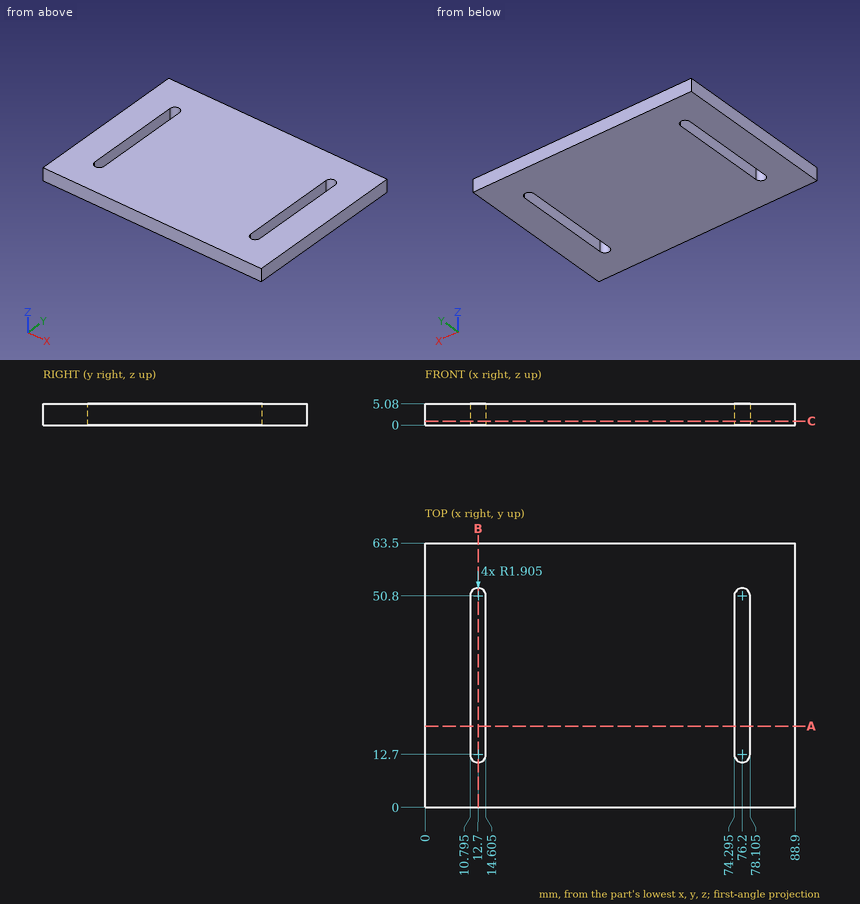
Check sheet for the drawn part. Datum: minimum x, y, z corner. Units: mm. Coordinates: 2 decimals unless noted, no trailing zeros. Loops run counter-clockwise (first coordinate to the right, second up) from the corner with the lowest first, then second, coordinate; pieces in that order, holes last. Notation, with made-up numbers: (25.5, -10.75) -> (72.5, -10.75) arc R32 cw to (72.5, 22.25) -> close; hole circle Ø10 at (5.25, 2). An arc over 180 degrees is marked (long way). Answer in a Markdown table with one row per item.
1. Sectioned sample at B-B, the plane x = 12.7. Record the boundary of the cut face in (y, z) (3 decimals), then the cut area to 3 significant figures.
Check values:
| item | result |
|---|---|
| outline | (0, 0) -> (10.795, 0) -> (10.795, 5.08) -> (0, 5.08) -> close; (52.705, 0) -> (63.5, 0) -> (63.5, 5.08) -> (52.705, 5.08) -> close |
| area | 110 mm2 |
2. Sectioned sample at C-C, the plane z = 0.95. Record the boundary of the cut face in (x, y) (3 decimals), then the cut area to 3 significant figures.
Check values:
| item | result |
|---|---|
| outline | (0, 0) -> (88.9, 0) -> (88.9, 63.5) -> (0, 63.5) -> close; hole (10.795, 12.7) arc R1.905 ccw to (14.605, 12.7) -> (14.605, 50.8) arc R1.905 ccw to (10.795, 50.8) -> close; hole (74.295, 12.7) arc R1.905 ccw to (78.105, 12.7) -> (78.105, 50.8) arc R1.905 ccw to (74.295, 50.8) -> close |
| area | 5,330 mm2 |
3. Sectioned sample at A-A, the plane y = 19.5. Record the boundary of the cut face in (x, z) (3 decimals).
Check values:
| item | result |
|---|---|
| outline | (0, 0) -> (10.795, 0) -> (10.795, 5.08) -> (0, 5.08) -> close; (14.605, 0) -> (74.295, 0) -> (74.295, 5.08) -> (14.605, 5.08) -> close; (78.105, 0) -> (88.9, 0) -> (88.9, 5.08) -> (78.105, 5.08) -> close |
4. Material ranges on line 1 along X through (y, z) = (33, 1.2) (3 decimals); line 2 along X through (y, z) = (52, 3.3), recorded low to high. Write a range as [from, to].
Check values:
| item | result |
|---|---|
| line 1 | x = [0, 10.795], [14.605, 74.295], [78.105, 88.9] |
| line 2 | x = [0, 11.22], [14.18, 74.72], [77.68, 88.9] |
